The model under review builds one solid part; all positions refer to its coordinate system, in mm. A direction names the side the tool comes from. Round coordinates to 2 decimals unless told otherwise and drop trailing zeros. Write each loop counter-clockwise with the first axis right and the second up, starting at its lowest first coordinate (ties: lowest second). Pieces come first, ordered by that corner, then holes.
Item 1: To check wall thickness, follow L1, parallel to Y at x = 0.95, z = 0.75; L2, parallel to Z at x = -1.3, y = 1.5; L3, parallel to Y at x = -0.1, z = 2.5. State the ranges of each line that lie inside material, in increasing order.
Item 2: Add section A-A (y = -1). Give the boundary of the cut face in (x, z), plus the area to 3 significant figures.
Item 3: Clearance check with a flat-ended pin moving along its axis: pin 1 Ø1.1 at (x, z) = (0, 1) entering from -Y. State where the tip first meets the part, or that it passes through.
Item 4: Draft analysis for pull direction X (two halves, no side actions). For faces 1 (the face through (0, 0.025, -1)), 2 (the face through (-1.4, 3.4, 1.753)), 3 (the face through (1.753, 2, 0)), state which applies: +X half, -X half, draft (parallel to the pull), parting line (faces both ways), or undercut.
Item 5: Machinability: for faces 4 (the face through (-0.4, 1.7, 4.216)), 5 (the face through (1.4, 3.4, 1.753)), 6 (the face through (-1.753, 2, 0)), which of the approach directions +Z, -Z, +X, -X, +Y, -Y give a long, thin tool a straight path to every point of the face, cutting with its end or side? Answer none if there is none.
Item 6: Add section C-C (z = 3.5). Give the boundary of the cut face in (x, y).
```python
from build123d import *

# Parameters (mm, degrees)
SKETCH1_W           = 3.5052
SKETCH1_H           = 3.5052
BOSS_EXTRUDE1_DEPTH = 3.81
SKETCH2_R           = 1.7526
BOSS_EXTRUDE2_DEPTH = 4.7498
SKETCH3_R           = 0.381
SKETCH3_W           = 0.508
SKETCH3_H           = 0.508
BOSS_EXTRUDE3_DEPTH = 2.9972
CUT_EXTRUDE2_START  = -0.0254
SKETCH4_R           = 1.27
SKETCH4_R_2         = 0.381
CUT_EXTRUDE2_DEPTH  = 0.0254
SKETCH5_R           = 1.6256
SKETCH5_R_2         = 0.381
CUT_EXTRUDE3_DEPTH  = 2.286
SKETCH6_R           = 0.66675


with BuildPart() as part:
    # Sketch1 → Boss-Extrude1 (new body)
    with BuildSketch(Plane(origin=(0, 0, 0), x_dir=(1, 0, 0), z_dir=(0, 1, 0))):
        Rectangle(SKETCH1_W, SKETCH1_H)
    extrude(amount=BOSS_EXTRUDE1_DEPTH)

    # Sketch2 → Boss-Extrude2 (add)
    with BuildSketch(Plane.XY.offset(1.7526)):
        with Locations((0, 2.0574)):
            Circle(SKETCH2_R)
    extrude(amount=BOSS_EXTRUDE2_DEPTH)

    # Sketch3 → Boss-Extrude3 (add)
    with BuildSketch(Plane.XZ):
        with Locations(Location((0, 0, 0), (0, 0, 270))):
            Circle(SKETCH3_R)
        with Locations((-1.27, 1.27)):
            Rectangle(SKETCH3_W, SKETCH3_H)
        with Locations((1.27, 1.27)):
            Rectangle(SKETCH3_W, SKETCH3_H)
        with Locations((-1.27, -1.27)):
            Rectangle(SKETCH3_W, SKETCH3_H)
        with Locations((1.27, -1.27)):
            Rectangle(SKETCH3_W, SKETCH3_H)
    extrude(amount=BOSS_EXTRUDE3_DEPTH)

    # Sketch4 → Cut-Extrude2 (cut)
    with BuildSketch(Plane.XZ.offset(CUT_EXTRUDE2_START)):
        with Locations(Location((0, 0, 0), (0, 0, 270))):
            Circle(SKETCH4_R)
        with Locations(Location((0, 0, 0), (0, 0, 270))):
            Circle(SKETCH4_R_2, mode=Mode.SUBTRACT)
    extrude(amount=CUT_EXTRUDE2_DEPTH, mode=Mode.SUBTRACT)

    # Sketch5 → Cut-Extrude3 (cut)
    with BuildSketch(Plane.XY.offset(6.5024)):
        with Locations((0, 2.0574)):
            Circle(SKETCH5_R)
        with Locations((0, 2.0574)):
            Circle(SKETCH5_R_2, mode=Mode.SUBTRACT)
    extrude(amount=-CUT_EXTRUDE3_DEPTH, mode=Mode.SUBTRACT)

    # Sketch6 → Cut-Revolve1 (revolve, cut)
    with BuildSketch(Plane(origin=(0, 0, 0), x_dir=(0, 0, -1), z_dir=(1, 0, 0)), mode=Mode.PRIVATE) as cut_revolve1_sk:
        with Locations((-5.9944, 1.00965)):
            Circle(SKETCH6_R)
    revolve(cut_revolve1_sk.sketch.rotate(Axis((0, 2.0574, 9.059220752), (0, 0, -1)), 270), axis=Axis((0, 2.0574, 9.059220752), (0, 0, -1)), mode=Mode.SUBTRACT)


solid = part.part
```
Numbers:
1. L1: y = 0.03 to 3.81
1. L2: z = -1.75 to 4.22
1. L3: y = 0.31 to 3.81
2. outline: (-1.52, -1.52) - (-1.02, -1.52) - (-1.02, -1.02) - (-1.52, -1.02) - close; (-1.52, 1.02) - (-1.02, 1.02) - (-1.02, 1.52) - (-1.52, 1.52) - close; circle Ø0.76 at (0, 0); (1.02, -1.52) - (1.52, -1.52) - (1.52, -1.02) - (1.02, -1.02) - close; (1.02, 1.02) - (1.52, 1.02) - (1.52, 1.52) - (1.02, 1.52) - close
2. area: 1.49 mm2
3. pin 1: stops at y = 0
4. face 1: undercut
4. face 2: draft
4. face 3: +X half
5. face 4: +Z
5. face 5: +Z, +X, +Y
5. face 6: +Z, -Z, -X, +Y, -Y
6. outline: circle Ø3.51 at (0, 2.06)
